Input: part model. Units: mm. Frame: model coordinates. Give positions to 0.01 mm unless a question says otherwise; leave off trailing zeros. Order: outer loops, then holes, each group sorted by start corner. A loop starts at its lowest first (then second) coordinate and runs counter-clockwise, first axis right, second up. Notation, with made-up numbers: (80.5, -24.5) - (117.5, -24.5) arc R18 ccw to (117.5, -13.5) - close; hole circle Ø9 at (54.5, 51.25). An arc over 180 degrees is marked (long way). Use a Markdown table: item, result.
from build123d import *

# Parameters (mm, degrees)
F0_W     = 55
F0_H     = 8
F1_DEPTH = 70
F2_R     = 6.35
F3_R     = 5.08


with BuildPart() as f1:
    # F0 (on Front) → F1 (new body)
    with BuildSketch(Plane.XZ):
        Rectangle(F0_W, F0_H)
    extrude(amount=F1_DEPTH)

    # F2
    f2_edges = [f1.edges().sort_by_distance(p)[0] for p in [
        (-27.5, -70, 0),
        (27.5, -70, 0),
        (27.5, 0, 0),
        (-27.5, 0, 0),
    ]]
    fillet(f2_edges, radius=F2_R)

    # F3
    f3_edges = [f1.edges().sort_by_distance(p)[0] for p in [
        (27.5, -35, 4),
        (25.640128, -1.859872, 4),
        (25.640128, -68.140128, 4),
        (0, 0, 4),
        (0, -70, 4),
        (-25.640128, -1.859872, 4),
        (-25.640128, -68.140128, 4),
        (-27.5, -35, 4),
    ]]
    fillet(f3_edges, radius=F3_R)


solid = f1.part
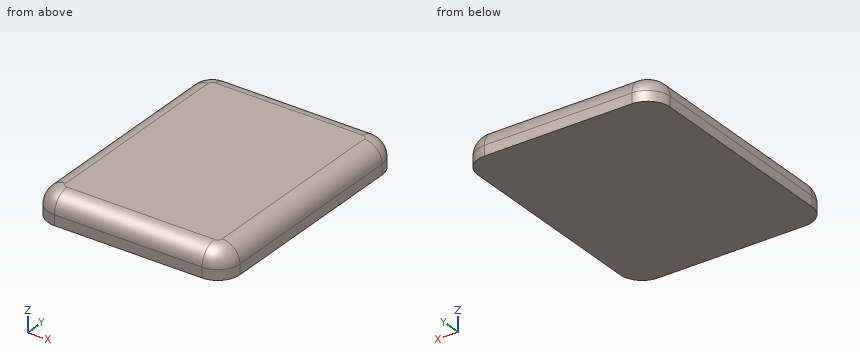
1. Pin query (flat end, axial travel): pin 1 (2 mm diameter, centred on y = -51, z = 1.5, fed in from -X); pin 2 (4 mm diameter, centred on x = 16, z = 1.5, fed in from +Y). Return the tip coordinate at first contact, or that it passes through.
Response:
| item | result |
|---|---|
| pin 1 | stops at x = -27.25 |
| pin 2 | stops at y = -0.03 |
2. Section query B-B (x = 0.5). Return loops of the section in (y, z), then the cut area to 3 significant figures.
Response:
| item | result |
|---|---|
| outline | (-70, -4) - (0, -4) - (0, -1.08) arc R5.08 ccw to (-5.08, 4) - (-64.92, 4) arc R5.08 ccw to (-70, -1.08) - close |
| area | 549 mm^2 |
3. Section query A-A (y = -23). Return loops of the section in (x, z).
Response:
| item | result |
|---|---|
| outline | (-27.5, -4) - (27.5, -4) - (27.5, -1.08) arc R5.08 ccw to (22.42, 4) - (-22.42, 4) arc R5.08 ccw to (-27.5, -1.08) - close |
4. Material intervals for line 1 along Y through (x, z) = (9, -1); line 2 along X through (y, z) = (-17, -1); line 3 along Y through (x, z) = (9.5, 1.25), sorted ascending.
Response:
| item | result |
|---|---|
| line 1 | y = -70 to 0 |
| line 2 | x = -27.5 to 27.5 |
| line 3 | y = -69.43 to -0.57 |
